Geometry: final body of the model. Coordinates: model frame, mm. Face numbers are marked on the shaded views. A direction names the side the tool comes from. Coordinates: 2 decimals unless noted, no trailing zeros. Write each loop counter-clockwise with the first axis right and the second up, starting at its lowest first coordinate (ties: lowest second). Pieces come first, ordered by that corner, then holes. Notation, with made-up numbers: (84, -0.5) -> (118, -0.5) arc R25 ccw to (118, 25.5) -> close; hole circle Ø3 at (48.25, -33.75). An arc over 180 degrees is marked (long way). One line per item, written item: value.
```python
from build123d import *

# Parameters (mm, degrees)
CYLINDER_R                  = 1.1
CYLINDER_DEPTH              = 10
CYLINDER001_R               = 1.1
CYLINDER001_DEPTH           = 10
SKETCH002_W                 = 23.3
SKETCH002_H                 = 12.5
PAD002_DEPTH                = 19.5
SKETCH_W                    = 32.5
SKETCH_H                    = 12.5
PAD001_DEPTH                = 4.5
SKETCH001_W                 = 36.061928
SKETCH001_H                 = 25.639376
PAD_DEPTH                   = 14
CUT002_PLACEMENT_ANGLE      = 180
CYLINDER010_R               = 3.6
CYLINDER010_DEPTH           = 8
CYLINDER010_ROLL_ANGLE      = 89.941329
CYLINDER010_PITCH_ANGLE     = 3.606623
CYLINDER010_PLACEMENT_ANGLE = -0.059115
PAD013_DEPTH                = 3
CYLINDER006_R               = 5
CYLINDER006_DEPTH           = 4
BOX_W                       = 71
BOX_H                       = 4
BOX_DEPTH                   = 14


with BuildPart() as cylinder:
    # Cylinder → Cylinder (new body)
    with BuildSketch(Plane(origin=(30, 22, 6), x_dir=(1, 0, 0), z_dir=(0, -1, 0))):
        Circle(CYLINDER_R)
    extrude(amount=CYLINDER_DEPTH)


with BuildPart() as obj1:
    # Cylinder001 → Cylinder001 (new body)
    with BuildSketch(Plane(origin=(2.2, 22, 6), x_dir=(1, 0, 0), z_dir=(0, -1, 0))):
        Circle(CYLINDER001_R)
    extrude(amount=CYLINDER001_DEPTH)

    # Fusion: union Cylinder
    add(cylinder.part)


with BuildPart() as cortecuerpo:
    # Sketch002 → Pad002 (new body)
    with BuildSketch(Plane.XZ):
        with Locations((16.4, 6.25)):
            Rectangle(SKETCH002_W, SKETCH002_H)
    extrude(amount=PAD002_DEPTH)


with BuildPart() as cortecuerpo_1:
    # Body004 placement: moved
    add(cortecuerpo.part.moved(Location((0, 19, 0))))


with BuildPart() as cortetornillos:
    # Sketch → Pad001 (new body)
    with BuildSketch(Plane.XZ):
        with Locations((16.25, 6.25)):
            Rectangle(SKETCH_W, SKETCH_H)
    extrude(amount=PAD001_DEPTH)


with BuildPart() as cortetornillos_1:
    # Body003 placement: moved
    add(cortetornillos.part.moved(Location((0, 23, 0))))


with BuildPart() as soporteservocaja:
    # Sketch001 → Pad (new body)
    with BuildSketch(Plane.XY):
        with Locations((15.881367, 9.413649)):
            Rectangle(SKETCH001_W, SKETCH001_H)
    extrude(amount=PAD_DEPTH)


with BuildPart() as soporteservocaja_1:
    # Body placement: moved
    add(soporteservocaja.part.moved(Location((0, 0, -1))))

    # Cut: cut CorteTornillos
    add(cortetornillos_1.part, mode=Mode.SUBTRACT)

    # Cut001: cut CorteCuerpo
    add(cortecuerpo_1.part, mode=Mode.SUBTRACT)

    # Cut002: cut obj1
    add(obj1.part, mode=Mode.SUBTRACT)


with BuildPart() as soporteservocaja_2:
    # Cut002 placement: moved
    add(soporteservocaja_1.part.moved(Location((-28.8, 27, 12))).rotate(Axis((-28.8, 27, 12), (1, 0, 0)), CUT002_PLACEMENT_ANGLE))


with BuildPart() as cylinder010:
    # Cylinder010 → Cylinder010 (new body)
    with BuildSketch(Plane.XY):
        Circle(CYLINDER010_R)
    extrude(amount=CYLINDER010_DEPTH)


with BuildPart() as cylinder010_1:
    # Cylinder010 roll: moved
    add(cylinder010.part.rotate(Axis((0, 0, 0), (1, 0, 0)), CYLINDER010_ROLL_ANGLE))


with BuildPart() as cylinder010_2:
    # Cylinder010 pitch: moved
    add(cylinder010_1.part.rotate(Axis((0, 0, 0), (0, 1, 0)), CYLINDER010_PITCH_ANGLE))


with BuildPart() as cylinder010_3:
    # Cylinder010 placement: moved
    add(cylinder010_2.part.moved(Location((21, 34, 6.3))).rotate(Axis((21, 34, 6.3), (0, 0, 1)), CYLINDER010_PLACEMENT_ANGLE))


with BuildPart() as obj2:
    # Sketch013 → Pad013 (new body)
    with BuildSketch(Plane.XZ):
        with BuildLine():
            ThreePointArc((-18.00002, 2), (-20, 0), (-18.00002, -2))
            Line((-18.00002, -2), (-2.073587, -3.25))
            ThreePointArc((-2.073587, -3.25), (0, -3.854383), (2.073587, -3.25))
            Line((2.073587, -3.25), (18.00002, -2))
            ThreePointArc((18.00002, -2), (20, 0), (18.00002, 2))
            Line((2.073587, 3.25), (18.00002, 2))
            ThreePointArc((2.073587, 3.25), (0, 3.862152), (-2.073587, 3.25))
            Line((-18.00002, 2), (-2.073587, 3.25))
        make_face()
    extrude(amount=PAD013_DEPTH)


with BuildPart() as obj2_1:
    # Body015 placement: moved
    add(obj2.part.moved(Location((21, 35, 6.3))))

    # Fusion009: union Cylinder010
    add(cylinder010_3.part)


with BuildPart() as cylinder006:
    # Cylinder006 → Cylinder006 (new body)
    with BuildSketch(Plane(origin=(-20, 35, 6), x_dir=(-1, 0, 0), z_dir=(0, -1, 0))):
        Circle(CYLINDER006_R)
    extrude(amount=CYLINDER006_DEPTH)


with BuildPart() as fusion010:
    # Box → Box (new body)
    with BuildSketch(Plane(origin=(-32, 29, -1), x_dir=(1, 0, 0), z_dir=(0, 0, 1))):
        with Locations((35.5, 2)):
            Rectangle(BOX_W, BOX_H)
    extrude(amount=BOX_DEPTH)

    # Cut011: cut Cylinder006
    add(cylinder006.part, mode=Mode.SUBTRACT)

    # Cut012: cut obj2
    add(obj2_1.part, mode=Mode.SUBTRACT)

    # Fusion010: union SoporteServoCaja
    add(soporteservocaja_2.part)


solid = fusion010.part
```
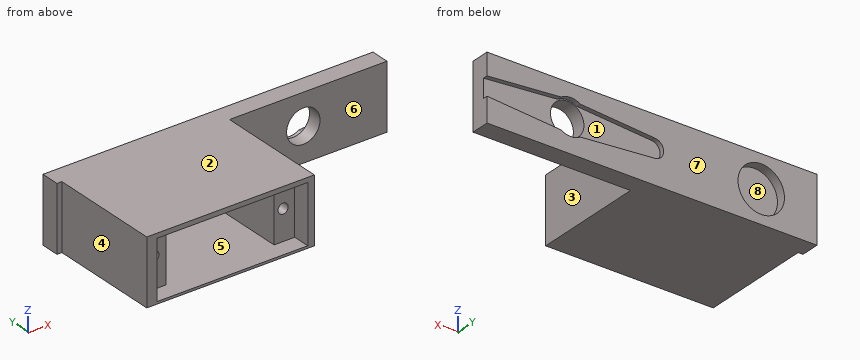
(1) Line query: line 1 (X direction, y = 31.55, z = 6); line 2 (X direction, y = 11.5, z = 7.5); line 3 (Z direction, x = 1.2, y = 11.5). Output: solid intervals per line, ascending. Write a range as [from, to].
Responses:
line 1: x = [-32, -25], [-15, 17.41], [24.58, 39]
line 2: x = [-30.95, -24.05], [-0.75, 5.11]
line 3: z = [-1, 4.9], [7.1, 13]
(2) Section C-C (y = 26.75). Return the cut outline in (x, z), then the cut area to 3 significant figures.
Responses:
outline: (-30.95, -1) -> (5.11, -1) -> (5.11, 13) -> (-30.95, 13) -> close; hole (-24.05, -0.5) -> (-0.75, -0.5) -> (-0.75, 12) -> (-24.05, 12) -> close
area: 214 mm2
(3) Pull-direction query (Z, two-part tool) for the marked faces 1, 2 and 3; classes: released by +Z, released by -Z, zero draft, split by the parting line, or undercut.
Responses:
face 1: undercut
face 2: released by +Z
face 3: zero draft
(4) Section A-A (y = 13.75). Return the cut outline in (x, z), then the cut area to 3 significant figures.
Responses:
outline: (-30.95, -1) -> (5.11, -1) -> (5.11, 13) -> (-30.95, 13) -> close; hole circle Ø2.2 at (-26.6, 6); hole (-24.05, -0.5) -> (-0.75, -0.5) -> (-0.75, 12) -> (-24.05, 12) -> close; hole circle Ø2.2 at (1.2, 6)
area: 206 mm2
(5) Section B-B (x = -20). Return the cut outline in (y, z).
Responses:
outline: (4.77, -1) -> (33, -1) -> (33, 1) -> (31, 1) -> (31, 11) -> (33, 11) -> (33, 13) -> (4.77, 13) -> (4.77, 12) -> (27.5, 12) -> (27.5, -0.5) -> (4.77, -0.5) -> close
(6) Reachability of the marked faces 4, 5, 6, 7 and 8 from +Z, -Z, +X, -X, +Y, -Y: full face, straight path, thin tool, end or side. Return the list, or none.
Responses:
face 4: +Z, -Z, -X, -Y
face 5: -Y
face 6: +Z, -Z, +X, -Y
face 7: +Z, -Z, +X, -X, +Y
face 8: +Y
(7) First-contact query: pin 1 (4 mm diameter, centred on y = 6, z = 8.5, fed in from +X); pin 2 (1.9 mm diameter, centred on y = 7.5, z = 5.5, fed in from -X); pin 3 (6 mm diameter, centred on x = 15.5, z = 5, fed in from +Y); pin 4 (2.5 mm diameter, centred on x = 1.5, z = 5.5, fed in from -Y). Flat tips, straight axial feed; report the tip coordinate or a pass-through.
Responses:
pin 1: stops at x = 5.11
pin 2: stops at x = -30.95
pin 3: stops at y = 33
pin 4: stops at y = 8.5
(8) Section D-D (x = 12.5). Return the cut outline in (y, z).
Responses:
outline: (29, -1) -> (33, -1) -> (33, 3.55) -> (32, 3.55) -> (32, 9.05) -> (33, 9.05) -> (33, 13) -> (29, 13) -> close
